Design review of the part built by this model. Coordinates are the model's own, in mm. Face numbers are marked on the shaded views. Coordinates: 2 decimals unless noted, no trailing zeros. Loops run counter-clockwise (first coordinate to the right, second up) from the corner with the lowest first, then second, coordinate; pieces in that order, holes last. Notation, with made-up numbers: (17.25, -5.75) -> (69.25, -5.75) arc R27 ccw to (69.25, 12.25) -> close; hole circle Ø6 at (81.25, 0). An arc over 180 degrees is marked (long way). One line per item, written item: value. Start each with the question number.
1. For probe 1 along Y at (x, z) = (0, 0); probe 2 along Z at (x, y) = (34.5, 3); probe 3 along Y at (x, z) = (28, -2), list the stretches that pass through material, from the lowest coordinate up.
2. Insertion check: pin 1 (8 mm diameter, centred on x = 20.5, z = 11, fed in from -Y); pin 2 (5 mm diameter, centred on x = 19, z = 4.5, fed in from +Y); pin 3 (22 mm diameter, centred on y = 0, z = 0, fed in from -X); pin 4 (3 mm diameter, centred on x = 8.5, y = -11, fed in from -Z). Each pin has a flat end and moves straight along its axis. Give the tip position at first contact, or say it passes through.
3. Draft analysis for pull direction Y (two halves, no side actions). For the marked faces 1 and 2, state which applies: pulls with the +Y half, pulls with the -Y half, needs draft (parallel to the pull), parting line crosses it, or undercut.
4. Add section C-C on x = 63. Write out the cut boundary in (y, z).
5. Add section A-A on z = 0. Write out the cut boundary in (x, y), plus the area to 3 significant figures.
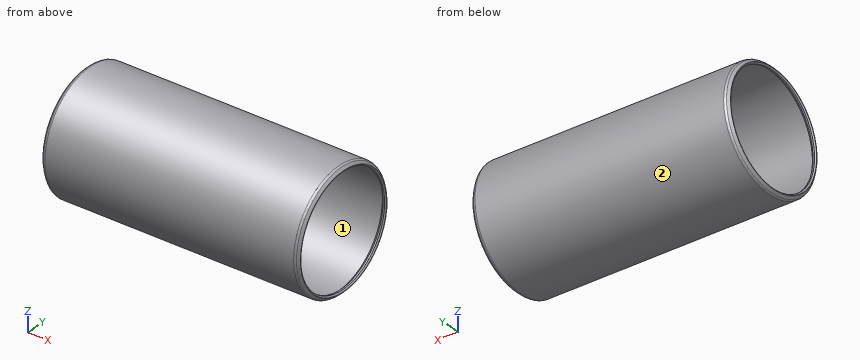
```python
from build123d import *


with BuildPart() as part:
    # Sketch1 → Revolve1 (revolve)
    with BuildSketch(Plane.XY, mode=Mode.PRIVATE) as revolve1_sk:
        with BuildLine():
            Line((-0.882617928, 18.554667928), (-0.508, 18.18005))
            Line((-0.508, 18.18005), (0, 18.18005))
            Line((0, 18.18005), (1.016, 19.19605))
            Line((1.016, 19.19605), (82.7913, 19.19605))
            Line((82.7913, 19.19605), (83.8073, 18.18005))
            Line((83.8073, 18.18005), (84.3153, 18.18005))
            Line((84.3153, 18.18005), (84.689917928, 18.554667928))
            ThreePointArc((84.689917928, 18.554667928), (84.727115367, 18.64447049), (84.689917928, 18.734273051))
            Line((84.689917928, 18.734273051), (83.95422049, 19.46997049))
            ThreePointArc((83.95422049, 19.46997049), (83.624606367, 19.690211605), (83.2358, 19.76755))
            Line((83.2358, 19.76755), (0.5715, 19.76755))
            ThreePointArc((0.5715, 19.76755), (0.182693633, 19.690211605), (-0.14692049, 19.46997049))
            Line((-0.14692049, 19.46997049), (-0.882617928, 18.734273051))
            ThreePointArc((-0.882617928, 18.734273051), (-0.919815367, 18.64447049), (-0.882617928, 18.554667928))
        make_face()
    revolve(revolve1_sk.sketch.rotate(Axis((83.8073, 0, 0), (-1, 0, 0)), 270), axis=Axis((83.8073, 0, 0), (-1, 0, 0)))


solid = part.part
```
Worked answers:
1. probe 1: y = -19.59 to -18.18, 18.18 to 19.59
1. probe 2: z = -19.54 to -18.96, 18.96 to 19.54
1. probe 3: y = -19.67 to -19.09, 19.09 to 19.67
2. pin 1: stops at y = -18.49
2. pin 2: stops at y = 19.67
2. pin 3: passes through
2. pin 4: stops at z = -17.34
3. face 1: undercut
3. face 2: parting line crosses it
4. outline: circle Ø39.54 at (0, 0); hole circle Ø38.39 at (0, 0)
5. outline: (-0.88, -18.73) -> (-0.15, -19.47) arc R1.02 ccw to (0.57, -19.77) -> (83.24, -19.77) arc R1.02 ccw to (83.95, -19.47) -> (84.69, -18.73) arc R0.13 ccw to (84.69, -18.55) -> (84.32, -18.18) -> (83.81, -18.18) -> (82.79, -19.2) -> (1.02, -19.2) -> (0, -18.18) -> (-0.51, -18.18) -> (-0.88, -18.55) arc R0.13 ccw to start; (-0.88, 18.55) -> (-0.51, 18.18) -> (0, 18.18) -> (1.02, 19.2) -> (82.79, 19.2) -> (83.81, 18.18) -> (84.32, 18.18) -> (84.69, 18.55) arc R0.13 ccw to (84.69, 18.73) -> (83.95, 19.47) arc R1.02 ccw to (83.24, 19.77) -> (0.57, 19.77) arc R1.02 ccw to (-0.15, 19.47) -> (-0.88, 18.73) arc R0.13 ccw to start
5. area: 101 mm²
